from build123d import *

# Parameters (mm, degrees)
ESQUISSE1_W                       = 40
ESQUISSE1_H                       = 15
BOSS_EXTRU_2_DEPTH                = 5
DIAM_TRE_DU_PER_AGE_5_0_5_1_D     = 5
DIAM_TRE_DU_PER_AGE_5_0_5_2_D     = 5
BOSS_EXTRU_3_DEPTH                = 40
ESQUISSE1_8_W                     = 5
ESQUISSE1_8_H                     = 20
BOSS_EXTRU_4_DEPTH                = 20
ESQUISSE1_9_W                     = 5
ESQUISSE1_9_H                     = 20
BOSS_EXTRU_5_DEPTH                = 20
DIAM_TRE_DU_PER_AGE_5_0_5_7_D     = 5
DIAM_TRE_DU_PER_AGE_5_0_5_7_DEPTH = 5
DIAM_TRE_DU_PER_AGE_5_0_5_8_D     = 5
DIAM_TRE_DU_PER_AGE_5_0_5_8_DEPTH = 5
ESQUISSE30_W                      = 40
ESQUISSE30_H                      = 20
ENL_V_MAT_EXTRU_1_DEPTH           = 35
DIAM_TRE_DU_PER_AGE_5_0_5_10_D    = 5
ESQUISSE37_W                      = 3
ESQUISSE37_H                      = 10
BOSS_EXTRU_6_DEPTH                = 10
ESQUISSE37_5_W                    = 3
ESQUISSE37_5_H                    = 10
ESQUISSE37_5_H_2                  = 10.219733904
BOSS_EXTRU_7_DEPTH                = 10
ENL_V_MAT_EXTRU_4_DEPTH           = 11
ENL_V_MAT_EXTRU_4_DEPTH_BACK      = 3
ENL_V_MAT_EXTRU_5_DEPTH           = 29.638558357
ENL_V_MAT_EXTRU_5_DEPTH_BACK      = 3
ENL_V_MAT_EXTRU_6_DEPTH           = 48
ENL_V_MAT_EXTRU_6_DEPTH_BACK      = 3


with BuildPart() as part:
    # Esquisse1 → Boss.-Extru.2 (new body)
    with BuildSketch(Plane.XY):
        with Locations((3.171437827, -12.450210199)):
            Rectangle(ESQUISSE1_W, ESQUISSE1_H)
    extrude(amount=BOSS_EXTRU_2_DEPTH)

    # Diamètre du perçage Ø5.0 (5)1 (through all)
    with Locations(Plane.XY.offset(5)):
        with Locations((13.171437827, -9.950210199)):
            Hole(DIAM_TRE_DU_PER_AGE_5_0_5_1_D / 2)

    # Diamètre du perçage Ø5.0 (5)2 (through all)
    with Locations(Plane.XY.offset(5)):
        with Locations((-6.828562173, -9.950210199)):
            Hole(DIAM_TRE_DU_PER_AGE_5_0_5_2_D / 2)

    # Esquisse1<6> → Boss.-Extru.3 (add)
    with BuildSketch(Plane.XY):
        Polygon((-16.828562173, 20.049789801), (23.171437827, 20.049789801), (28.171437827, 20.049789801), (33.171437827, 20.049789801), (33.171437827, -4.950210199), (23.171437827, -4.950210199), (-16.828562173, -4.950210199), (-26.828562173, -4.950210199), (-26.828562173, 20.049789801), (-21.828562173, 20.049789801), align=None)
    extrude(amount=BOSS_EXTRU_3_DEPTH)

    # Esquisse1<8> → Boss.-Extru.4 (add)
    with BuildSketch(Plane.XY):
        with Locations((25.671437827, 10.049789801)):
            Rectangle(ESQUISSE1_8_W, ESQUISSE1_8_H)
    extrude(amount=-BOSS_EXTRU_4_DEPTH)

    # Esquisse1<9> → Boss.-Extru.5 (add)
    with BuildSketch(Plane.XY):
        with Locations((-19.328562173, 10.049789801)):
            Rectangle(ESQUISSE1_9_W, ESQUISSE1_9_H)
    extrude(amount=-BOSS_EXTRU_5_DEPTH)

    # Diamètre du perçage Ø5.0 (5)7
    with Locations(Plane(origin=(28.171437827, 0, 0), x_dir=(0, 0, -1), z_dir=(1, 0, 0))):
        with Locations((10, 10.049789801)):
            Hole(DIAM_TRE_DU_PER_AGE_5_0_5_7_D / 2, depth=DIAM_TRE_DU_PER_AGE_5_0_5_7_DEPTH)

    # Diamètre du perçage Ø5.0 (5)8
    with Locations(Plane.ZY.offset(21.828562173)):
        with Locations((-10, 10.049789801)):
            Hole(DIAM_TRE_DU_PER_AGE_5_0_5_8_D / 2, depth=DIAM_TRE_DU_PER_AGE_5_0_5_8_DEPTH)

    # Esquisse30 → Enlèv. mat.-Extru.1 (cut)
    with BuildSketch(Plane.XY.offset(40)):
        with Locations((3.171437827, 7.549789801)):
            Rectangle(ESQUISSE30_W, ESQUISSE30_H)
    extrude(amount=-ENL_V_MAT_EXTRU_1_DEPTH, mode=Mode.SUBTRACT)

    # Diamètre du perçage Ø5.0 (5)10 (through all)
    with Locations(Plane(origin=(33.171437827, 0, 0), x_dir=(0, 0, -1), z_dir=(1, 0, 0))):
        with Locations((-10, 7.549789801)):
            Hole(DIAM_TRE_DU_PER_AGE_5_0_5_10_D / 2)

    # Esquisse37 → Boss.-Extru.6 (add)
    with BuildSketch(Plane.XY.offset(5)):
        with Locations((-15.328562173, -9.950210199)):
            Rectangle(ESQUISSE37_W, ESQUISSE37_H)
    extrude(amount=BOSS_EXTRU_6_DEPTH)

    # Esquisse37<5> → Boss.-Extru.7 (add)
    with BuildSketch(Plane.XY.offset(5)):
        with Locations((-15.328562173, -9.950210199)):
            Rectangle(ESQUISSE37_5_W, ESQUISSE37_5_H)
        with Locations((21.671437827, -10.060077151)):
            Rectangle(ESQUISSE37_5_W, ESQUISSE37_5_H_2)
        with Locations((3.309996184, -9.950210199)):
            Rectangle(ESQUISSE37_5_W, ESQUISSE37_5_H)
    extrude(amount=BOSS_EXTRU_7_DEPTH)

    # Esquisse38 → Enlèv. mat.-Extru.4 (cut, two sides)
    with BuildSketch(Plane.ZY.offset(16.828562173)) as enl_v_mat_extru_4_sk:
        Polygon((15, -14.950210199), (15, -4.950210199), (5, -14.950210199), align=None)
    extrude(amount=ENL_V_MAT_EXTRU_4_DEPTH, mode=Mode.SUBTRACT)
    extrude(enl_v_mat_extru_4_sk.sketch, amount=-ENL_V_MAT_EXTRU_4_DEPTH_BACK, mode=Mode.SUBTRACT)

    # Esquisse40 → Enlèv. mat.-Extru.5 (cut, two sides)
    with BuildSketch(Plane.ZY.offset(-1.809996184)) as enl_v_mat_extru_5_sk:
        Polygon((15, -14.950210199), (15, -4.950210199), (5, -14.950210199), align=None)
    extrude(amount=ENL_V_MAT_EXTRU_5_DEPTH, mode=Mode.SUBTRACT)
    extrude(enl_v_mat_extru_5_sk.sketch, amount=-ENL_V_MAT_EXTRU_5_DEPTH_BACK, mode=Mode.SUBTRACT)

    # Esquisse41 → Enlèv. mat.-Extru.6 (cut, two sides)
    with BuildSketch(Plane.ZY.offset(-20.171437827)) as enl_v_mat_extru_6_sk:
        Polygon((15, -15.169944103), (15, -4.950210199), (5, -15.169944103), align=None)
    extrude(amount=ENL_V_MAT_EXTRU_6_DEPTH, mode=Mode.SUBTRACT)
    extrude(enl_v_mat_extru_6_sk.sketch, amount=-ENL_V_MAT_EXTRU_6_DEPTH_BACK, mode=Mode.SUBTRACT)


solid = part.part
Can you work these out from the model? Positions are in its coordinate system, mm. A direction names the side the tool comes from. Coordinates: 2 decimals unless noted, no trailing zeros. Order: outer loops, then holes, each group sorted by start corner. A loop starts at its lowest first (then second) coordinate and runs counter-clockwise, first axis right, second up. Notation, with made-up numbers: (67, 70) - (114, 70) arc R10 cw to (114, 84) - close; hole circle Ø4 at (80, 33). An arc over 180 degrees is marked (long way). Answer as a JSON object with one key per item and string values. Group by question number.
Q1. Imagine slicing it at D-D (y = 3). Please give me the cut outline in (x, z), and give its area (3 significant figures).
Q2. Imagine slicing it at C-C (x = -11). Please give me the cut outline in (y, z).
Q3. I need wall thicknesses on line 1 (Y direction, x = 30, z = 10); line 2 (Y direction, x = -14, z = 26); line 3 (X direction, y = 17.5, z = 11.5). Which ranges of each line are inside material? Lowest first, please. Write a range as from..to.
Q4. Will these pins go through, and if not, where does the flat tip stop? P1, Ø4, axis at y = -8, z = 10, coming from the +X side; P2, Ø10, axis at x = 4, y = -2, coming from the -Z side; P3, Ø8, axis at y = -2.5, z = -4.5, coming from the +X side; P4, Ø4, axis at y = 9.5, z = 11, coming from the -X side.
Q5. We'd pull the mould along X, two halves only. Please class faces 4 (the face through (4, 20.05, 16)), 5 (the face through (1.81, -8, 8)), 6 (the face through (28.171, 8, -8)), 7 (the face through (15.014, -8.261, 2.465)): +X half, -X half, draft (parallel to the pull), parting line (faces both ways), or undercut.
Q6. Imagine slicing it at A-A (z = -10). Please give me the cut outline in (x, y), and give its area (3 significant figures).
Q7. Imagine slicing it at B-B (z = 32.5). Please give me the cut outline in (x, y), and give its area (3 significant figures).
Q8. On a 3-axis mill with a long thin cutter (end or side, diameter ignored), from which of +Z, -Z, +X, -X, +Y, -Y can I reach the whole of each face in a straight line? I mean faces 1 (the face through (-16.829, -11, 4)), 2 (the face through (3, -4.95, 20)), 3 (the face through (26, 0.05, -10)). Say none if no direction works.
Determined:
{
 "1": {"outline": "(-26.83, 0) - (-21.83, 0) - (-21.83, -20) - (-16.83, -20) - (-16.83, 0) - (23.17, 0) - (23.17, -20) - (28.17, -20) - (28.17, 0) - (33.17, 0) - (33.17, 40) - (23.17, 40) - (23.17, 5) - (-16.83, 5) - (-16.83, 40) - (-26.83, 40) - close", "area": "1,200 mm2"},
 "2": {"outline": "(-19.95, 0) - (20.05, 0) - (20.05, 40) - (17.55, 40) - (17.55, 5) - (-2.45, 5) - (-2.45, 40) - (-4.95, 40) - (-4.95, 5) - (-19.95, 5) - close"},
 "3": {"line 1": "y = -4.95..5.05, 10.05..20.05", "line 2": "y = -4.95..-2.45, 17.55..20.05", "line 3": "x = -26.83..-16.83, 23.17..33.17"},
 "4": {"P1": "stops at x = 23.17", "P2": "stops at z = 0", "P3": "stops at x = 28.17", "P4": "stops at x = -26.83"},
 "5": {"face 4": "draft", "face 5": "undercut", "face 6": "+X half", "face 7": "undercut"},
 "6": {"outline": "(-21.83, 0.05) - (-16.83, 0.05) - (-16.83, 7.55) - (-21.83, 7.55) - close; (-21.83, 12.55) - (-16.83, 12.55) - (-16.83, 20.05) - (-21.83, 20.05) - close; (23.17, 0.05) - (28.17, 0.05) - (28.17, 7.55) - (23.17, 7.55) - close; (23.17, 12.55) - (28.17, 12.55) - (28.17, 20.05) - (23.17, 20.05) - close", "area": "150 mm2"},
 "7": {"outline": "(-26.83, -4.95) - (33.17, -4.95) - (33.17, 20.05) - (-26.83, 20.05) - close; hole (-16.83, -2.45) - (23.17, -2.45) - (23.17, 17.55) - (-16.83, 17.55) - close", "area": "700 mm2"},
 "8": {"face 1": "+Z, -Z, -X, -Y", "face 2": "+Z, -Y", "face 3": "-Z, +X, -X, -Y"}
}
